Autodesk Inventor part; units mm, degrees
ref_plane "YZ Plane" through (0, 0, 0) normal (1, 0, 0) x (0, 1, 0)
ref_plane "XZ Plane" through (0, 0, 0) normal (0, 1, 0) x (-1, 0, 0)
ref_plane "XY Plane" through (0, 0, 0) normal (0, 0, 1) x (1, 0, 0)
sketch "Sketch1" plane through (0, 0, 0) normal (0, 1, 0) x (-1, 0, 0)
  circle A0 centre (0, 0) radius 6.35
  circle A1 centre (0, 0) radius 7.9375
  line L0 (5.5563, 15.875) -> (-5.5563, 15.875)
  line L1 (-5.5563, 15.875) -> (-5.5563, -15.875)
  line L2 (-5.5563, -15.875) -> (5.5563, -15.875)
  line L3 (5.5563, -15.875) -> (5.5563, 15.875)
  line L4 (5.5563, 15.875) -> (-5.5563, -15.875) construction
  line L5 (-5.5563, 15.875) -> (5.5563, -15.875) construction
  line L6 (-5.5563, 0) -> (5.5563, 0) construction
  line L7 (-5.5563, 15.875) -> (5.5563, 15.875)
  line L8 (5.5563, 15.875) -> (5.5563, 11.1125)
  line L9 (5.5563, 11.1125) -> (-5.5563, 11.1125)
  line L10 (-5.5563, 11.1125) -> (-5.5563, 15.875)
  line L11 (-5.5563, 13.4937) -> (5.5563, 13.4937) construction
  circle A2 centre (-3.175, 13.4937) radius 1.4732
  line L12 (0, 15.875) -> (0, 11.1125) construction
  circle A3 centre (3.175, 13.4937) radius 1.4732
  line L13 (5.5563, -15.875) -> (-5.5563, -15.875)
  line L14 (-5.5563, -15.875) -> (5.5563, -15.875)
  line L15 (5.5563, -15.875) -> (5.5563, -11.1125)
  line L16 (5.5563, -11.1125) -> (-5.5563, -11.1125)
  line L17 (-5.5563, -11.1125) -> (-5.5563, -15.875)
  line L18 (-5.5563, -13.4937) -> (5.5563, -13.4937) construction
  circle A4 centre (-3.175, -13.4937) radius 1.4732
  line L19 (0, -15.875) -> (0, -11.1125) construction
  circle A5 centre (3.175, -13.4937) radius 1.4732
  circle A6 centre (0, 0) radius 4.7625
  point P0 (-5.5563, 5.6685)
  point P1 (-5.5563, -5.6685)
  point P2 (5.5563, -5.6685)
  point P3 (5.5563, 5.6685)
  dimension "d0" = 12.7
  dimension "d1" = 15.875
  dimension "d2" = 11.1125
  dimension "d3" = 31.75
  dimension "d4" = 4.7625
  dimension "d5" = 2.9464
  dimension "d6" = 2.3813
  dimension "d7" = 9.525
extrude "Extrusion1" add sketch "Sketch1" against normal blind 1.5875
extrude "Extrusion2" add sketch "Sketch1" against normal blind 6.35 contours A0 L3 A1 | A0 L1 A1 L3 | L3 A1 L1 A0 | A0 L1 A1 | A1 L1 L9 L3 | L3 L16 L1 A1
fillet "Fillet1" radius 3.175 4 edges at (-5.5563, -3.175, 5.6685) (-5.5563, -3.175, -5.6685) (5.5563, -3.175, 5.6685) (5.5563, -3.175, -5.6685)
sketch "Sketch2" plane through (0, -6.35, 0) normal (0, -1, 0) x (1, 0, 0)
  circle A0 centre (0, 0) radius 6.9453
  dimension "d13" = 13.8906
properties part number "Shaft Brace" material "Aluminum 6061"
Design review of the part built by this model. Coordinates are the model's own, in mm. A direction names the side the tool comes from. Give positions to 0.01 mm unless a question says otherwise; leave off trailing zeros. Write each loop counter-clockwise with the first axis right and the second up, starting at its lowest first coordinate (ties: lowest second). Pieces come first, ordered by that corner, then holes. Notation, with made-up numbers: M -13.75,37 L -7.75,37 A29 cw -7.75,60 Z; hole C 74.5,13.5 d1. An arc over 180 degrees is marked long. Answer as a JSON object with one key per item and string values. Group by question number.
1) Tool access review of faces 1 (the face through (5.556, -2, 9)), 2 (the face through (-1, -1.588, 5)), 3 (the face through (0, -1.588, -13)): name each direction out of +Z, -Z, +X, -X, +Y, -Y from which nothing blocks a thin tool from reaching the whole face with its end or side.
2) We need section D-D (x = 3.75). Count the separate pieces of the cut face and the enclosed holes in it, and give its area (3 significant figures).
3) Mouldability with a two-part tool opening along Z and no side actions: class faces 4 (the face through (0, -1, 15.875)), 5 (the face through (5.556, -2, -9)), 6 (the face through (3.494, -0.783, 12.056)), 7 (the face through (0, -1, -15.875)) as released by +Z, released by -Z, zero draft, split by the parting line, or undercut.
4) For line 1 along Z through (x, y) = (0, -5.2); line 2 along Z through (x, y) = (0, -1) (1 decimal); line 3 along X through (y, z) = (-2.5, 9.5), list the stretches that pass through material, from the lowest coordinate up.
5) Clearance check with flat-ended pins moving along their axes: pin 1 Ø1.5 at (y, z) = (-5, -10) entering from +X; pin 2 Ø2.5 at (x, z) = (-3.18, -13.49) entering from -Y; pin 3 Ø3 at (x, y) = (5.5, -5.5) entering from -Z; pin 4 Ø3.5 at (x, z) = (3.18, -13.49) entering from -Y. State where each tip first meets the part, or that it passes through.
6) We need section A-A (z = 0). Give the boundary of the cut face in (x, y).
Answer key:
{
 "1": {"face 1": "+Z, +X, +Y, -Y", "face 2": "-Y", "face 3": "-Z, +X, -X, -Y"},
 "2": {"separate pieces": "4", "enclosed holes": "0", "area": "89.5 mm²"},
 "3": {"face 4": "released by +Z", "face 5": "zero draft", "face 6": "undercut", "face 7": "released by -Z"},
 "4": {"line 1": "z = -11.11 to -6.35, 6.35 to 11.11", "line 2": "z = -15.9 to -4.8, 4.8 to 15.9", "line 3": "x = -5.56 to 5.56"},
 "5": {"pin 1": "stops at x = 5.56", "pin 2": "passes through", "pin 3": "stops at z = -11.11", "pin 4": "stops at y = -1.59"},
 "6": {"outline": "M -7.94,-6.35 L -6.35,-6.35 L -6.35,-1.59 L -4.76,-1.59 L -4.76,0 L -7.94,0 Z; M 4.76,-1.59 L 6.35,-1.59 L 6.35,-6.35 L 7.94,-6.35 L 7.94,0 L 4.76,0 Z"}
}
